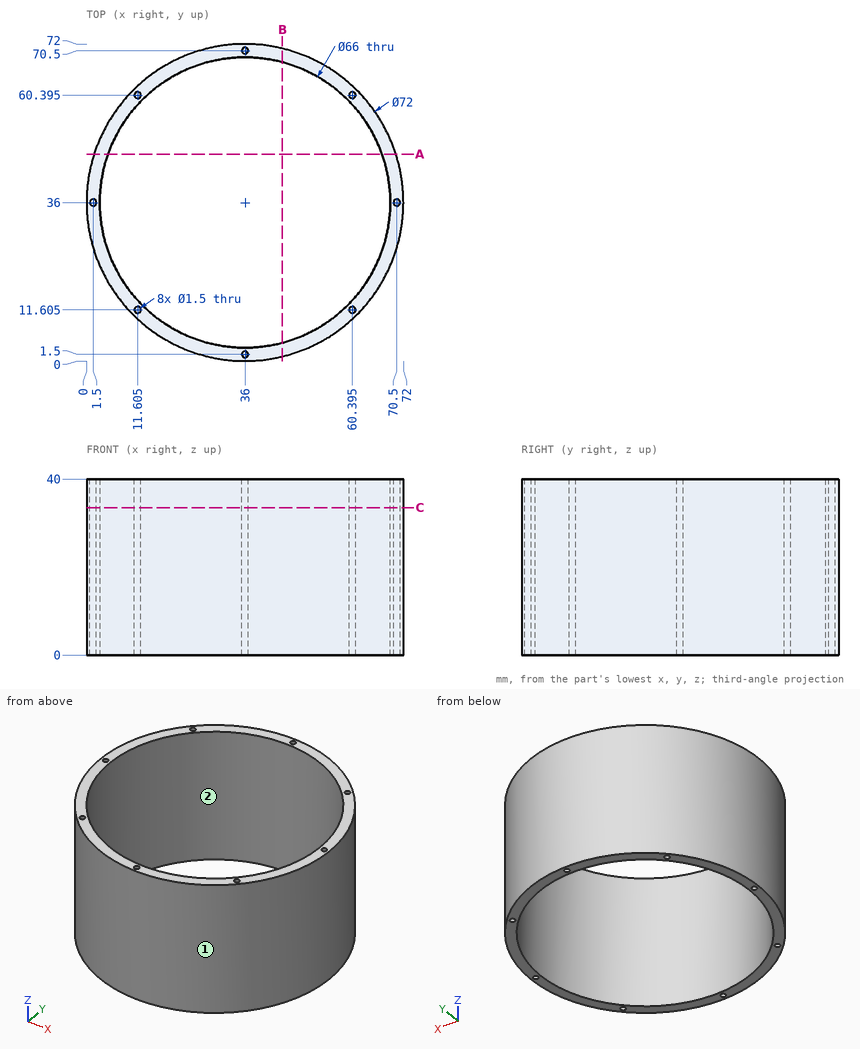
The figure shows three views and two pictorial views of one solid part (mm, origin at its lowest corner). Answer the questions. Coordinates: 2 decimals unless noted, no trailing zeros. Loops run counter-clockwise (first coordinate to the right, second up) from the corner with the lowest first, then second, coordinate; pieces in that order, holes last.
1) Determine the mould class of the marked faces 1 and 2 for opening direction Y: pulls with the +Y half, pulls with the -Y half, needs draft (parallel to the pull), parting line crosses it, or undercut.
2) Find the intervals of material crossed by L1, parallel to Y at x = 36, z = 26; L2, parallel to Y at x = 60, z = 2.5; L3, parallel to Y at x = 62, z = 36, in increasing order.
3) Find section B-B on x = 44.5. Write down the section's boundary in (y, z).
4) Find section C-C on z = 33.5. Give the number of separate pieces and of enclosed holes in the cut face, then the cut area to 3 significant figures.
5) Find section A-A on y = 47. Write down the section's boundary in (x, z).
6) Flat-ended cylindrical pins translate along their axes: pin 1 Ø2.5 at (x, y) = (36, 1.5) entering from +Z; pin 2 Ø0.9 at (x, y) = (11.6, 60.4) entering from -Z; pin 3 Ø4 at (y, z) = (58, 33) entering from +X; pin 4 Ø6 at (x, z) = (59.5, 20.5) entering from -Y. Find the tip coordinate at first contact, or state that the pin passes through.
Values:
1. face 1: parting line crosses it
1. face 2: undercut
2. L1: y = 0 to 0.75, 2.25 to 3, 69 to 69.75, 71.25 to 72
2. L2: y = 9.17 to 10.97, 12.24 to 13.35, 58.65 to 59.76, 61.03 to 62.83
2. L3: y = 11.1 to 15.68, 56.32 to 60.9
3. outline: (1.02, 0) - (4.11, 0) - (4.11, 40) - (1.02, 40) - close; (67.89, 0) - (70.98, 0) - (70.98, 40) - (67.89, 40) - close
4. separate pieces: 1
4. enclosed holes: 9
4. area: 636 mm2
5. outline: (1.72, 0) - (4.89, 0) - (4.89, 40) - (1.72, 40) - close; (67.11, 0) - (70.28, 0) - (70.28, 40) - (67.11, 40) - close
6. pin 1: stops at z = 40
6. pin 2: passes through
6. pin 3: stops at x = 65.93
6. pin 4: stops at y = 6.41
